Could you check a few things on this drawing? It's one solid part, dimensions in mm from its lowest x, y, z. Give positions to 0.01 mm unless a question says otherwise; leave off trailing zeros. Order: outer loops, then holes, each group sorted by start corner. A loop starts at its lowest first (then second) coordinate and runs counter-clockwise, first axis right, second up.
Item 1: I'm going to push flat-ended pins straight in: pin 1 Ø1 at (x, z) = (28.5, 4.5) entering from -Y; pin 2 Ø3 at (y, z) = (22, 4) entering from +X; pin 3 Ø2 at (x, z) = (16, 4.5) entering from -Y. Where does each tip first touch, or does it pass through?
Item 2: I want a section at A-A, the plane y = 34. Write out the boundary of the cut face in (x, z).
Item 3: I want a section at C-C, the plane z = 2. Write out the boundary of the cut face in (x, y), then the cut area to 3 significant figures.
Item 4: If I drill on line 1 along X through (y, z) = (33.5, 3.5); line 2 along X through (y, z) = (31.5, 4.75); line 3 along Y through (x, z) = (30.5, 2.25), over which ranges is the centre line in solid material (lowest first)?
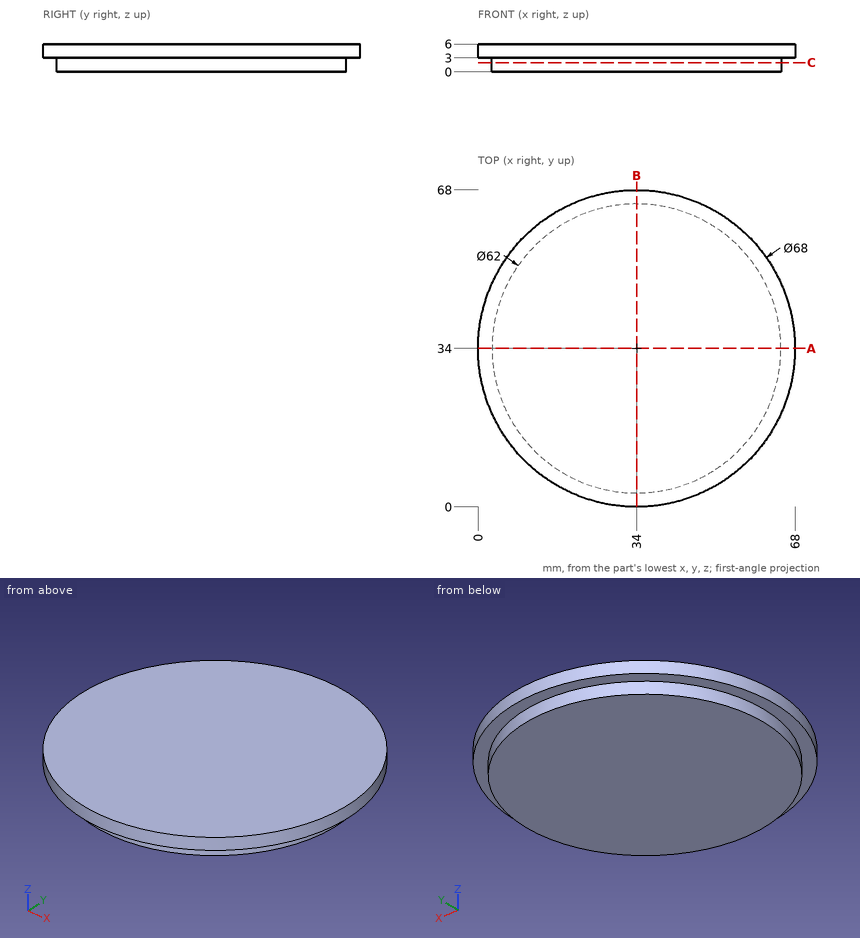
Results list:
1. pin 1: stops at y = 0.37
1. pin 2: stops at x = 66.34
1. pin 3: stops at y = 4.56
2. outline: (0, 3) - (3, 3) - (3, 0) - (65, 0) - (65, 3) - (68, 3) - (68, 6) - (0, 6) - close
3. outline: circle Ø62 at (34, 34)
3. area: 3,020 mm2
4. line 1: x = 0 to 68
4. line 2: x = 0.09 to 67.91
4. line 3: y = 3.2 to 64.8
